Can you work these out from the drawing? Everything is in mm from the part's minimum corner. A direction names the side the tool comes from. Round coordinates to 2 decimals unless told otherwise and drop trailing zeros. Answer as CSV lines item,"result".
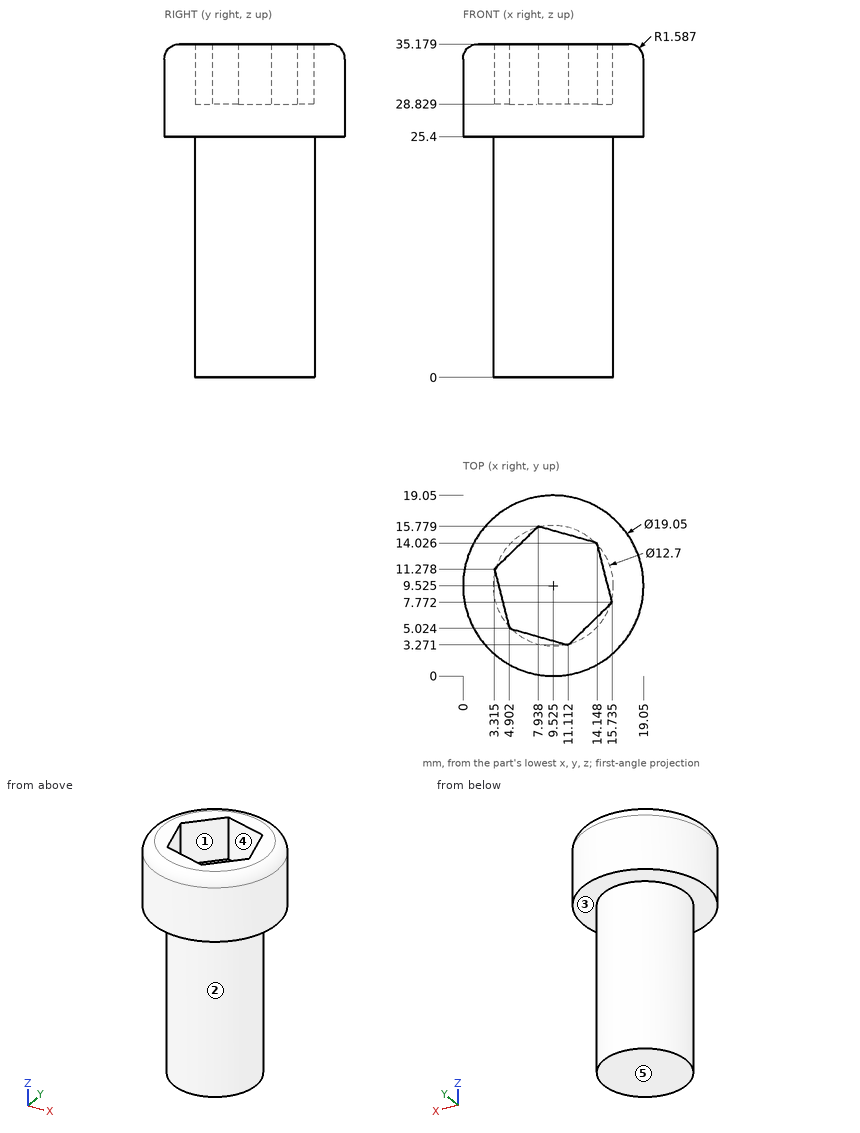
Item 1: Will these pins go through, and if not, where does the flat tip stop? pin 1 (5 mm diameter, centred on x = 6, z = 28.5, fed in from +Y) (1 decimal); pin 2 (1 mm diameter, centred on x = 15.5, z = 27, fed in from +Y); pin 3 (5 mm diameter, centred on x = 13, z = 18.5, fed in from -Y); pin 4 (10 mm diameter, centred on y = 8, z = 24, fed in from -X).
Results found:
pin 1,"stops at y = 19"
pin 2,"stops at y = 17.32"
pin 3,"stops at y = 3.25"
pin 4,"stops at x = 0"
Item 2: For the marked faces 4 and 5, which set-ups out of +Z, -Z, +X, -X, +Y, -Y let a thin tool reach every point of the face, with its end or its side?
Results found:
face 4,"+Z"
face 5,"-Z, +X, -X, +Y, -Y"
Item 3: If we mould it in two halves opening along Y, with no side actions, what happens to the marked faces 1, 2 and 3? For each: pulls with the +Y half, pulls with the -Y half, needs draft (parallel to the pull), parting line crosses it, or undercut.
Results found:
face 1,"undercut"
face 2,"parting line crosses it"
face 3,"needs draft"
Item 4: I need wall thicknesses on L1, parallel to Z at x = 11.75, y = 15.75; L2, parallel to Z at x = 7, y = 11.75; L3, parallel to Y at x = 11.25, z = 13.5 (1 decimal). Which ranges of each line are inside material? Lowest first, please.
Results found:
L1,"z = 25.4 to 35.18"
L2,"z = 0 to 28.83"
L3,"y = 3.4 to 15.6"
